Part model, mm, in its own coordinate system. A direction names the side the tool comes from. Give positions to 0.01 mm unless a question says otherwise; leave off trailing zeros. Loops run counter-clockwise (first coordinate to the right, second up) from the corner with the lowest first, then second, coordinate; pieces in that order, holes last. Notation, with made-up numbers: (62.25, 10.25) -> (91.25, 10.25) arc R34 ccw to (91.25, 47.25) -> close; hole circle Ø1 at (83.25, -8.75). An arc over 180 degrees is marked (long way). One line per question, with ' | ' between items.
```python
from build123d import *

# Parameters (mm, degrees)
SKETCH1_R           = 29.845
BOSS_EXTRUDE1_DEPTH = 17.78
SKETCH2_R           = 8.89
BOSS_EXTRUDE2_DEPTH = 4.2418
SKETCH3_R           = 7.493
BOSS_EXTRUDE3_DEPTH = 4.064
SKETCH4_R           = 8.255
BOSS_EXTRUDE4_DEPTH = 0.762
SKETCH6_R           = 0.95
CUT_EXTRUDE1_DEPTH  = 25.4


with BuildPart() as part:
    # Sketch1 → Boss-Extrude1 (new body)
    with BuildSketch(Plane(origin=(0, 0, 0), x_dir=(1, 0, 0), z_dir=(0, 1, 0))):
        Circle(SKETCH1_R)
    extrude(amount=BOSS_EXTRUDE1_DEPTH)

    # Sketch2 → Boss-Extrude2 (add)
    with BuildSketch(Plane(origin=(0, 17.78, 0), x_dir=(1, 0, 0), z_dir=(0, 1, 0))):
        Circle(SKETCH2_R)
    extrude(amount=BOSS_EXTRUDE2_DEPTH)

    # Sketch3 → Boss-Extrude3 (add)
    with BuildSketch(Plane(origin=(0, 0, 0), x_dir=(-1, 0, 0), z_dir=(0, -1, 0))):
        Circle(SKETCH3_R)
    extrude(amount=BOSS_EXTRUDE3_DEPTH)

    # Sketch4 → Boss-Extrude4 (add)
    with BuildSketch(Plane.XZ.offset(4.064)):
        Circle(SKETCH4_R)
    extrude(amount=BOSS_EXTRUDE4_DEPTH)

    # Sketch6 → Cut-Extrude1 (cut)
    with BuildSketch(Plane(origin=(0, -4.826, 0), x_dir=(-1, 0, 0), z_dir=(0, -1, 0))):
        with BuildLine():
            Line((-2.33826859, -1.35), (2.33826859, -1.35))
            ThreePointArc((2.33826859, -1.35), (2.7, 0), (2.33826859, 1.35))
            Line((2.33826859, 1.35), (-2.33826859, 1.35))
            ThreePointArc((-2.33826859, 1.35), (-2.7, 0), (-2.33826859, -1.35))
        make_face()
        Circle(SKETCH6_R, mode=Mode.SUBTRACT)
    extrude(amount=-CUT_EXTRUDE1_DEPTH, mode=Mode.SUBTRACT)


solid = part.part
```
1) Pull direction X, two halves, no side cores. Call faces 4 (the flat face through (0, 22.022, 0)), 5 (the cylindrical face through (-1.93, 19.87, 8.68)), 6 (the cylindrical face through (-2.7, 7.7, 0)): pulls with the +X half, pulls with the -X half, needs draft (parallel to the pull), parting line crosses it, or undercut.
Found:
face 4: needs draft | face 5: parting line crosses it | face 6: undercut
2) Pin check, flat tips, straight feed: P1, Ø4, axis at x = 21.5, y = 8, coming from the -Z side; P2, Ø12, axis at x = 1, y = 18.5, coming from the +Z side (3 decimals); P3, Ø2, axis at x = 6, y = 11.5, coming from the +Z side. Stop position of each tip, or through.
Found:
P1: z = -22.59 | P2: z = 29.845 | P3: z = 29.42
3) Drill centre lines: line 1 (Y direction, x = -16, z = 24); line 2 (X direction, y = 2.75, z = 21); line 3 (X direction, y = 10.5, z = -13). Where is each one in solid material? Low to high.
Found:
line 1: 0 to 17.78 | line 2: -21.21 to 21.21 | line 3: -26.86 to 26.86
4) Saw through at A-A (y = 5.5). Give the cut face in (x, z) (3 decimals).
Found:
outline: circle Ø59.69 at (0, 0); circle Ø1.9 at (0, 0); hole (-2.338, -1.35) -> (2.338, -1.35) arc R2.7 ccw to (2.338, 1.35) -> (-2.338, 1.35) arc R2.7 ccw to start
5) Tool access for faces 1 (the cylindrical face through (2.7, 7.7, 0)), 2 (the flat face through (4, -4.064, -7)), 3 (the flat face through (6, 17.78, -7)): list every direction of +Z, -Z, +X, -X, +Y, -Y with a clear straight run to the whole face (end or side of a thin tool).
Found:
face 1: -Y | face 2: none | face 3: +Y
6) Saw through at C-C (x = 0). Give the cut face in (y, z) (3 decimals).
Found:
outline: (-4.826, -8.255) -> (-4.064, -8.255) -> (-4.064, -7.493) -> (0, -7.493) -> (0, -29.845) -> (17.78, -29.845) -> (17.78, -8.89) -> (22.022, -8.89) -> (22.022, 8.89) -> (17.78, 8.89) -> (17.78, 29.845) -> (0, 29.845) -> (0, 7.493) -> (-4.064, 7.493) -> (-4.064, 8.255) -> (-4.826, 8.255) -> (-4.826, 1.35) -> (20.574, 1.35) -> (20.574, 0.95) -> (-4.826, 0.95) -> (-4.826, -0.95) -> (20.574, -0.95) -> (20.574, -1.35) -> (-4.826, -1.35) -> close
7) Saw through at D-D (z = 6). Give the cut face in (x, y), and give its area (3 significant figures).
Found:
outline: (-29.24, 0) -> (-4.49, 0) -> (-4.49, -4.06) -> (-5.67, -4.06) -> (-5.67, -4.83) -> (5.67, -4.83) -> (5.67, -4.06) -> (4.49, -4.06) -> (4.49, 0) -> (29.24, 0) -> (29.24, 17.78) -> (6.56, 17.78) -> (6.56, 22.02) -> (-6.56, 22.02) -> (-6.56, 17.78) -> (-29.24, 17.78) -> close | area: 1,140 mm2
8) Saw through at B-B (z = 0). Give the cut face in (x, y) (3 decimals), and give its area (3 significant figures).
Found:
outline: (-29.845, 0) -> (-7.493, 0) -> (-7.493, -4.064) -> (-8.255, -4.064) -> (-8.255, -4.826) -> (-2.7, -4.826) -> (-2.7, 20.574) -> (-0.95, 20.574) -> (-0.95, -4.826) -> (0.95, -4.826) -> (0.95, 20.574) -> (2.7, 20.574) -> (2.7, -4.826) -> (8.255, -4.826) -> (8.255, -4.064) -> (7.493, -4.064) -> (7.493, 0) -> (29.845, 0) -> (29.845, 17.78) -> (8.89, 17.78) -> (8.89, 22.022) -> (-8.89, 22.022) -> (-8.89, 17.78) -> (-29.845, 17.78) -> close | area: 1,120 mm2
